Can you work these out from the drawing? Everything is in mm from the part's minimum corner. Round coordinates to 2 decimals unless told otherwise and drop trailing zeros. Write each loop counter-clockwise with the first axis right and the second up, starting at its lowest first coordinate (ties: lowest second). Pieces come first, ordered by that corner, then holes. Notation, with made-up numbers: (64, 50.5) -> (72, 50.5) arc R25 cw to (72, 70.5) -> close; hole circle Ø1 at (18, 66.5). An arc over 180 degrees is marked (long way). One line per question, with ' | ' between items. Start each with the question number.
1. If I drill on line 1 along X through (y, z) = (5.75, 9.75) (1 decimal); line 2 along X through (y, z) = (4.25, 4.25); line 3 along X through (y, z) = (6, 3) (1 decimal), over which ranges is the centre line in solid material (lowest first)? Write a range as [from, to].
2. Imagine slicing it at D-D, the plane y = 8. List the corners of the cut face in (x, z) for me.
3. Imagine slicing it at A-A, the plane x = 4.75. List the corners of the cut face in (y, z) for me.
4. Imagine slicing it at B-B, the plane x = 7.5. List the corners of the cut face in (y, z) for me.
5. Thinking about a two-plate mould opening in Y: for the marked faces 1, 2 and 3, which applies, released by +Y, released by -Y, zero draft, split by the parting line, or undercut?
6. Imagine slicing it at C-C, the plane z = 8. State how many separate pieces and enclosed holes the cut face has, and give its area (3 significant figures).
7. For pin 1 Ø2 at (x, y) = (5, 8.5) entering from -Z; pin 2 Ø1 at (y, z) = (8, 5.5) entering from -X; pin 3 Ø1.3 at (x, y) = (7.5, 5.76) entering from +Z, each with a flat end and sliding along its axis, tell me the tip position at first contact or that it passes through.
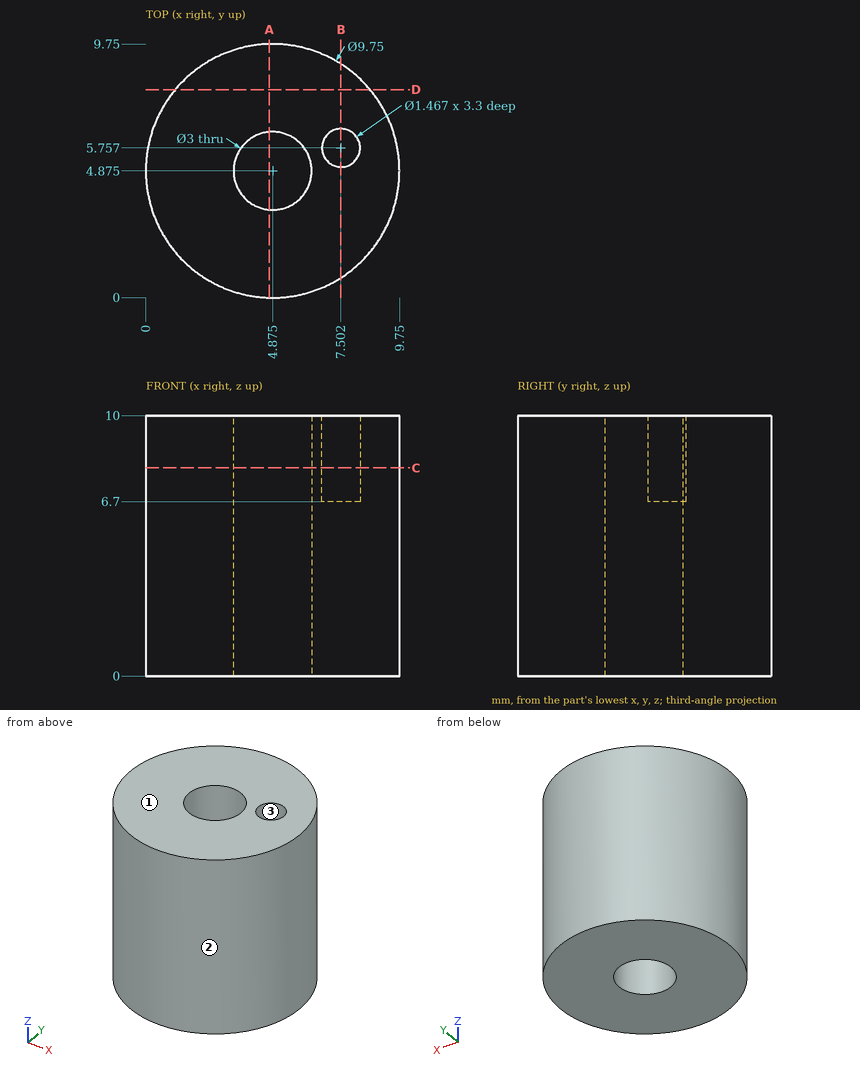
Geometry results:
1) line 1: x = [0.1, 3.7], [6.1, 6.8], [8.2, 9.7] | line 2: x = [0.04, 3.51], [6.24, 9.71] | line 3: x = [0.1, 3.9], [5.9, 9.6]
2) outline: (1.13, 0) -> (8.62, 0) -> (8.62, 10) -> (1.13, 10) -> close
3) outline: (0, 0) -> (3.38, 0) -> (3.38, 10) -> (0, 10) -> close; (6.37, 0) -> (9.75, 0) -> (9.75, 10) -> (6.37, 10) -> close
4) outline: (0.77, 0) -> (8.98, 0) -> (8.98, 10) -> (6.49, 10) -> (6.49, 6.7) -> (5.02, 6.7) -> (5.02, 10) -> (0.77, 10) -> close
5) face 1: zero draft | face 2: split by the parting line | face 3: undercut
6) separate pieces: 1 | enclosed holes: 2 | area: 65.9 mm2
7) pin 1: stops at z = 0 | pin 2: stops at x = 0.77 | pin 3: stops at z = 6.7
